Design review of the part shown in the three views and the two pictorial views. Dimensions are in mm from the part's minimum x, y and z. Coordinates: 2 decimals unless noted, no trailing zeros. Order: outer loops, then holes, each group sorted by start corner. A loop starts at its lowest first (then second) coordinate and runs counter-clockwise, first axis right, second up. Notation, with made-up numbers: (58.25, 74) -> (81.25, 74) arc R34 cw to (81.25, 113) -> close; hole circle Ø10 at (48.25, 20). An arc over 180 degrees is marked (long way). Answer as a JSON object with one key per item and string values. Group by question number.
1) Add section A-A, the plane x = 0.75. Write out the cut boundary in (y, z).
2) Add section B-B, the plane y = 1.5. Write out the cut boundary in (x, z), then the cut area to 4 significant figures.
3) Add section D-D, the plane x = 2.5. Write out the cut boundary in (y, z).
4) Wall thickness on L1, parallel to Z at x = 8, y = 1.45; L2, parallel to Z at x = 1.5, y = 0.7; L3, parallel to Y at x = 3.5, z = 0.7: over which ranges is each line inside the solid? List them lowest first.
5) Add section C-C, the plane z = 2.1. Write out the cut boundary in (x, y), then the cut area to 3 significant figures.
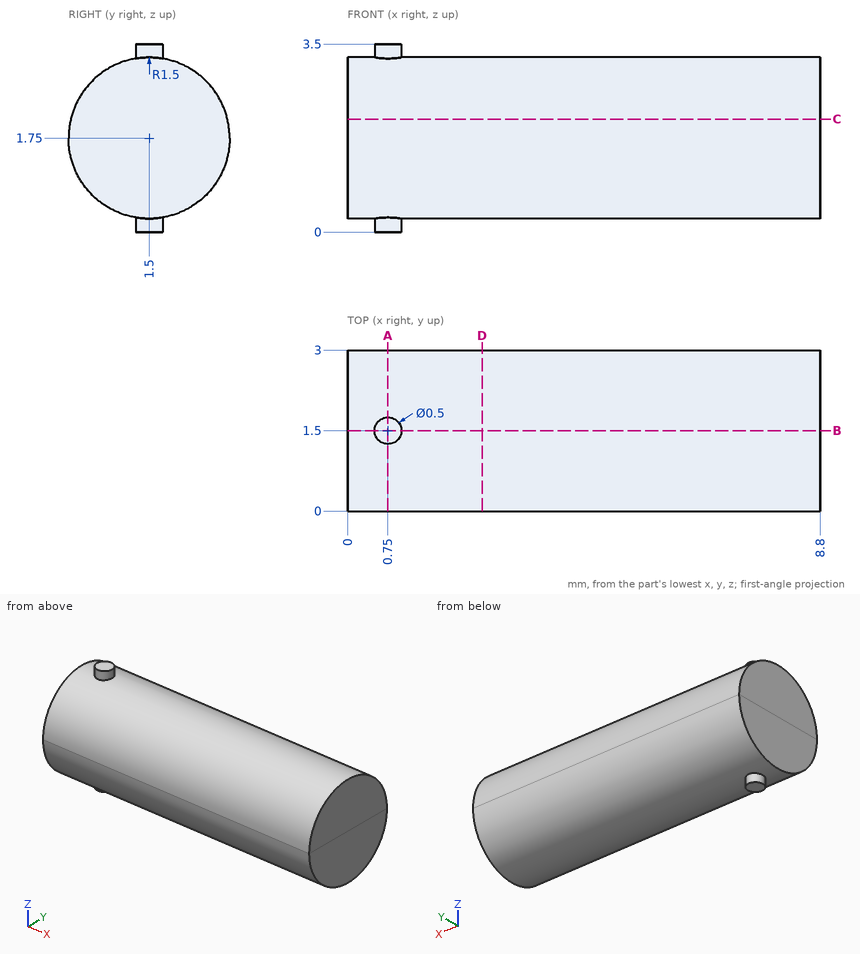
Output values:
{
 "1": {"outline": "(1.25, 0) -> (1.75, 0) -> (1.75, 0.27) arc R1.5 ccw to (1.75, 3.23) -> (1.75, 3.5) -> (1.25, 3.5) -> (1.25, 3.23) arc R1.5 ccw to (1.25, 0.27) -> close"},
 "2": {"outline": "(0, 0.25) -> (0.5, 0.25) -> (0.5, 0) -> (1, 0) -> (1, 0.25) -> (8.8, 0.25) -> (8.8, 3.25) -> (1, 3.25) -> (1, 3.5) -> (0.5, 3.5) -> (0.5, 3.25) -> (0, 3.25) -> close", "area": "26.65 mm²"},
 "3": {"outline": "circle Ø3 at (1.5, 1.75)"},
 "4": {"L1": "z = 0.25 to 3.25", "L2": "z = 0.48 to 3.02", "L3": "y = 0.43 to 2.57"},
 "5": {"outline": "(0, 0.04) -> (8.8, 0.04) -> (8.8, 2.96) -> (0, 2.96) -> close", "area": "25.7 mm²"}
}
